Verification items for the finished model (mm, model axes). Give positions to 0.01 mm unless a question says otherwise; leave off trailing zeros. Loops run counter-clockwise (first coordinate to the right, second up) from the corner with the lowest first, then second, coordinate; pieces in that order, holes last. Notation, with made-up numbers: (88, 50) - (146, 50) arc R21 cw to (146, 58) - close; hole circle Ø9 at (33.5, 9). An arc over 180 degrees is marked (long way). One line per item, written item: value. Start each with the question number.
1. Gauge pin test, flat ends, axial feed: pin 1 (3 mm diameter, centred on x = -11, y = 2, fed in from +Z); pin 2 (2 mm diameter, centred on x = 4.5, y = 1.5, fed in from -Z). Record the tip position at first contact, or that the pin passes through.
2. Scan lines: L1, parallel to X at y = 3.25, z = 25.4; L2, parallel to Z at x = -9, y = 5.75; L3, parallel to X at y = 3, z = 0. Record each from-to range of solid material in increasing order. Write a range as [from, to].
3. Sectioned sample at C-C (y = 3.5). Record the cut outline in (x, z) (1 decimal), plus the area to 3 significant figures.
4. Mould release check, pull along X, two halves, no side actions. Record for faces 1 (the cylindrical face through (-0.36, 3.13, 38.1)), 2 (the flat face through (12, 0, -9)), 3 (the cylindrical face through (-1.372, 3.131, -27.552)): pulls with the +X half, pulls with the -X half, needs draft (parallel to the pull), parting line crosses it, or undercut.
5. Sectioned sample at A-A (z = 25.4). Record the cut outline in (x, y), plus the area to 3 significant figures.
6. Sectioned sample at B-B (x = 0). Record the cut outline in (y, z).
7. Sectioned sample at D-D (x = -7). Record the cut outline in (y, z).
from build123d import *

# Parameters (mm, degrees)
SKETCH1_R              = 38.1
SKETCH1_R_2            = 14.3129
BOSS_EXTRUDE1_DEPTH    = 6.35
SKETCH4_OUTSIDE_W      = 99.79
SKETCH4_OUTSIDE_H      = 99.79
CUT_EXTRUDE1_DEPTH     = 55.254423783
F_10_CLEARANCE_HOLE2_D = 5.1054


with BuildPart() as part:
    # Sketch1 → Boss-Extrude1 (new body)
    with BuildSketch(Plane(origin=(0, 0, 0), x_dir=(1, 0, 0), z_dir=(0, 1, 0))):
        with Locations(Location((0, 0, 0), (0, 0, 270))):
            Circle(SKETCH1_R)
        with Locations(Location((0, 0, 0), (0, 0, 270))):
            Circle(SKETCH1_R_2, mode=Mode.SUBTRACT)
    extrude(amount=BOSS_EXTRUDE1_DEPTH)

    # Sketch4 outside → Cut-Extrude1 (cut, through all)
    with BuildSketch(Plane(origin=(0, 6.35, 0), x_dir=(1, 0, 0), z_dir=(0, 1, 0))):
        Rectangle(SKETCH4_OUTSIDE_W, SKETCH4_OUTSIDE_H)
        with BuildLine():
            Line((-25.4, -26.181720723), (-25.4, 26.181720723))
            ThreePointArc((-25.4, 26.181720723), (-24.922489894, 28.260246127), (-23.585714286, 29.92196654))
            ThreePointArc((-23.585714286, 29.92196654), (0, 38.1), (23.585714286, 29.92196654))
            ThreePointArc((23.585714286, 29.92196654), (24.922489894, 28.260246127), (25.4, 26.181720723))
            Line((25.4, 26.181720723), (25.4, -26.181720723))
            ThreePointArc((25.4, -26.181720723), (24.922489894, -28.260246127), (23.585714286, -29.92196654))
            ThreePointArc((23.585714286, -29.92196654), (0, -38.1), (-23.585714286, -29.92196654))
            ThreePointArc((-23.585714286, -29.92196654), (-24.922489894, -28.260246127), (-25.4, -26.181720723))
        make_face(mode=Mode.SUBTRACT)
    extrude(amount=-CUT_EXTRUDE1_DEPTH, mode=Mode.SUBTRACT)

    # #10 Clearance Hole2 (through all)
    with Locations(Plane(origin=(0, 6.35, 0), x_dir=(1, 0, 0), z_dir=(0, 1, 0))):
        with Locations((0, 25.4), (0, -25.4)):
            Hole(F_10_CLEARANCE_HOLE2_D / 2)


solid = part.part
Results are:
1. pin 1: stops at z = 36.9
1. pin 2: stops at z = -37.94
2. L1: x = [-25.4, -2.55], [2.55, 25.4]
2. L2: z = [-37.02, -11.13], [11.13, 37.02]
2. L3: x = [-25.4, -14.31], [14.31, 25.4]
3. outline: (-25.4, -26.2) arc R4.8 ccw to (-23.6, -29.9) arc R38.1 ccw to (23.6, -29.9) arc R4.8 ccw to (25.4, -26.2) - (25.4, 26.2) arc R4.8 ccw to (23.6, 29.9) arc R38.1 ccw to (-23.6, 29.9) arc R4.8 ccw to (-25.4, 26.2) - close; hole circle Ø28.6 at (0, 0); hole circle Ø5.1 at (0, -25.4); hole circle Ø5.1 at (0, 25.4)
3. area: 2,870 mm^2
4. face 1: parting line crosses it
4. face 2: needs draft
4. face 3: undercut
5. outline: (-25.4, 0) - (-2.55, 0) - (-2.55, 6.35) - (-25.4, 6.35) - close; (2.55, 0) - (25.4, 0) - (25.4, 6.35) - (2.55, 6.35) - close
5. area: 290 mm^2
6. outline: (0, -38.1) - (6.35, -38.1) - (6.35, -27.95) - (0, -27.95) - close; (0, -22.85) - (6.35, -22.85) - (6.35, -14.31) - (0, -14.31) - close; (0, 14.31) - (6.35, 14.31) - (6.35, 22.85) - (0, 22.85) - close; (0, 27.95) - (6.35, 27.95) - (6.35, 38.1) - (0, 38.1) - close
7. outline: (0, -37.45) - (6.35, -37.45) - (6.35, -12.48) - (0, -12.48) - close; (0, 12.48) - (6.35, 12.48) - (6.35, 37.45) - (0, 37.45) - close
